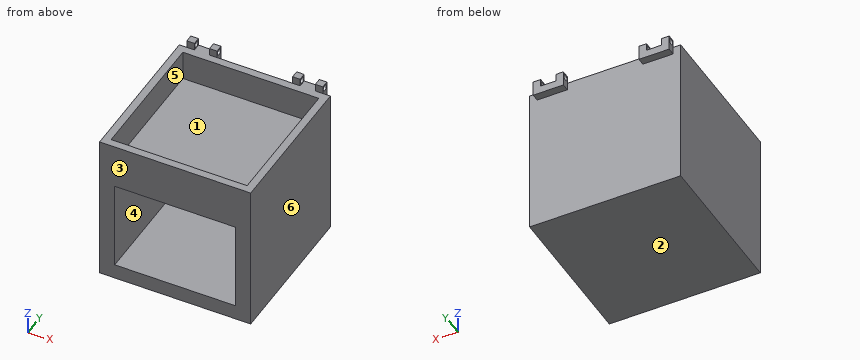
Autodesk Fusion 360 part; units mm, degrees
sketch "Sketch1" plane through (0, 0, 0) normal (0, 0, 1) x (1, 0, 0)
  line L0 (50, 50) -> (-50, 50)
  line L1 (-50, 50) -> (-50, -50)
  line L2 (-50, -50) -> (50, -50)
  line L3 (50, -50) -> (50, 50)
  line L4 (50, 50) -> (-50, -50) construction
  line L5 (-50, 50) -> (50, -50) construction
  dimension "d1" = 100
  dimension "d2" = 100
extrude "Extrude1" add sketch "Sketch1" along normal blind 100
sketch "Sketch2" plane through (0, 0, 100) normal (0, 0, 1) x (-1, 0, 0)
  line L0 (-50, 50) -> (-50, -50)
  line L1 (-50, -50) -> (50, -50)
  line L2 (50, -50) -> (50, 50)
  line L3 (50, 50) -> (-50, 50)
  line L4 (-45, -45) -> (45, -45)
  line L5 (45, -45) -> (45, 45)
  line L6 (45, 45) -> (-45, 45)
  line L7 (-45, 45) -> (-45, -45)
  line L8 (-45, -45) -> (45, 45) construction
  line L9 (45, -45) -> (-45, 45) construction
  dimension "d6" = 90
  dimension "d7" = 90
extrude "Extrude2" cut sketch "Sketch2" against normal blind 20 contours L4 L5 L6 L7
sketch "Sketch3" plane through (0, -50, 0) normal (0, -1, 0) x (1, 0, 0)
  line L0 (-50, 0) -> (50, 0)
  line L1 (50, 0) -> (50, 100)
  line L2 (50, 100) -> (-50, 100)
  line L3 (-50, 100) -> (-50, 0)
  line L4 (-40, 10) -> (-40, 40)
  line L5 (-40, 40) -> (40, 40)
  line L6 (40, 40) -> (40, 10)
  line L7 (40, 10) -> (-40, 10)
  line L8 (-40, 70) -> (40, 70)
  line L9 (40, 70) -> (40, 40)
  line L10 (-40, 40) -> (-40, 70)
extrude "Extrude3" cut sketch "Sketch3" against normal blind 90 contours L4 L5 L6 L7 | L5 L8 L9 L10
sketch "Sketch4" plane through (0, 0, 100) normal (0, 0, 1) x (-1, 0, 0)
  line L0 (45, -45) -> (-45, -45)
  line L1 (-45, -45) -> (-45, 45)
  line L2 (-45, 45) -> (45, 45)
  line L3 (45, 45) -> (45, -45)
  line L4 (-50, 50) -> (-50, -50)
  line L5 (-50, -50) -> (50, -50)
  line L6 (50, -50) -> (50, 50)
  line L7 (50, 50) -> (-50, 50)
  line L8 (45, -50) -> (45, -55)
  line L9 (-45, -50) -> (-45, -55)
  line L10 (-45, -55) -> (-25, -55)
  line L11 (-25, -55) -> (-25, -50)
  line L12 (45, -55) -> (25, -55)
  line L13 (25, -55) -> (25, -50)
  dimension "d12" = 5
  dimension "d13" = 5
  dimension "d14" = 20
  dimension "d15" = 20
extrude "Extrude4" add sketch "Sketch4" along normal mid plane 10 contours L5 L9 L10 L11 | L5 L8 L12 L13
sketch "Sketch5" plane through (0, 0, 105) normal (0, 0, 1) x (-1, 0, 0)
  line L0 (-45, -50) -> (-45, -55)
  line L1 (-45, -55) -> (-25, -55)
  line L2 (-25, -55) -> (-25, -50)
  line L3 (-25, -50) -> (-45, -50)
  line L4 (-25, -55) -> (-30, -55)
  line L5 (-30, -55) -> (-40, -55)
  line L6 (-40, -55) -> (-40, -50)
  line L7 (-30, -50) -> (-30, -55)
  line L8 (25, -55) -> (30, -55)
  line L9 (30, -55) -> (40, -55)
  line L10 (40, -55) -> (40, -50)
  line L11 (40, -50) -> (30, -50)
  line L12 (30, -50) -> (30, -55)
extrude "Extrude5" cut sketch "Sketch5" against normal blind 5 contours L1 L3 L5 L6 L7 | L9 L10 L11 L12
sketch "Sketch9" plane through (45, 0, 0) normal (1, 0, 0) x (0, 1, 0)
  line L0 (55, 95) -> (55, 105)
  line L1 (55, 105) -> (50, 105)
  line L2 (50, 105) -> (50, 100)
  line L3 (50, 100) -> (50, 95)
  line L4 (50, 95) -> (55, 95)
  circle A0 centre (52.5, 102.5) radius 2
extrude "Extrude7" cut sketch "Sketch9" against normal blind 130 contours A0
Verification items for the finished model (mm, model axes). Face numbers are marked on the shaded views. A direction names the side the tool comes from. Coordinates: 2 decimals unless noted, no trailing zeros. Order: outer loops, then holes, each group sorted by start corner. A loop starts at its lowest first (then second) coordinate and runs counter-clockwise, first axis right, second up. Notation, with made-up numbers: M -8,81.25 L 19,81.25 A15 ccw 19,106.25 Z; hole C 41,-3.5 d7. An arc over 180 degrees is marked long. One line per item, written item: value. Start each with the question number.
Item 1: Mould release check, pull along Y, two halves, no side actions. Record for the marked faces 1, 2 and 3: released by +Y, released by -Y, zero draft, split by the parting line, or undercut.
Item 2: Gauge pin test, flat ends, axial feed: pin 1 (5.5 mm diameter, centred on x = -28.5, z = 103, fed in from -Y); pin 2 (2.5 mm diameter, centred on y = 53.5, z = 102.5, fed in from -X); pin 3 (4 mm diameter, centred on x = -16.5, y = -24, fed in from +Z); pin 4 (5.5 mm diameter, centred on y = 51.5, z = 102, fed in from -X). Record the tip position at first contact, or that the pin passes through.
Item 3: Access from +Z, -Z, +X, -X, +Y, -Y to the whole of each face (thin tool, end or side, straight path). Record for the marked faces 4, 5 and 6.
Item 4: Sectioned sample at D-D (y = -30). Enter the section's corners in (x, z).
Item 5: Sectioned sample at A-A (z = 102.5). Count the separate pieces of the cut face and the enclosed holes in it, then the cut area to 3 significant figures.
Item 6: Scan lines: probe 1 along X at (y, z) = (-43, 24.5); probe 2 along Z at (x, y) = (37.5, 12); probe 3 along Z at (x, y) = (-41.7, 52.5). Record each from-to range of solid material in increasing order.
Item 7: Sectioned sample at C-C (x = 33). Enter the section's corners in (y, z), then the cut area to 4 significant figures.
Conclusion:
1. face 1: undercut
1. face 2: zero draft
1. face 3: released by -Y
2. pin 1: stops at y = 50
2. pin 2: stops at x = -45
2. pin 3: stops at z = 80
2. pin 4: stops at x = -50
3. face 4: -Y
3. face 5: +Z
3. face 6: +Z, -Z, +X, +Y, -Y
4. outline: M -50,0 L 50,0 L 50,100 L 45,100 L 45,80 L -45,80 L -45,100 L -50,100 Z; hole M -40,10 L 40,10 L 40,70 L -40,70 Z
5. separate pieces: 8
5. enclosed holes: 0
5. area: 20.0 mm^2
6. probe 1: x = -50 to -40, 40 to 50
6. probe 2: z = 0 to 10, 70 to 80
6. probe 3: z = 95 to 100.5, 104.5 to 105
7. outline: M -50,0 L 50,0 L 50,95 L 55,95 L 55,100 L 45,100 L 45,80 L -45,80 L -45,100 L -50,100 L -50,70 L 40,70 L 40,10 L -50,10 Z
7. area: 2,825 mm^2
